The model under review builds one solid part; all positions refer to its coordinate system, in mm. A direction names the side the tool comes from. Round coordinates to 2 decimals unless told otherwise and drop trailing zeros. Loops run counter-clockwise (first coordinate to the right, second up) from the corner with the lowest first, then second, coordinate; pieces in that order, holes last. Notation, with made-up numbers: M -16,-27 L 10,-27 A26 ccw 10,4 Z; hole C -15,21.5 d2. An arc over 180 degrees is marked long. Return JSON: item names as keys, results as strings. Group by question number.
Q1. For faces 4 (the face through (84.51, 2.75, 4.59)), 5 (the face through (1, 0, -1)), 6 (the face through (50.8, 3, -16)), list the 3-axis set-ups (+Z, -Z, +X, -X, +Y, -Y) from which the entire face can be reached by the end or side of a thin tool; tool diameter is ignored.
Q2. Clearance check with a flat-ended pin moving along its axis: pin 1 Ø0.8 at (x, z) = (76.2, 18.72) entering from +Y. State where the tip first meets the part, or that it passes through.
Q3. To check wall thickness, follow line 1 along X through (y, z) = (2.2, -15.5); line 2 along Z through (x, y) = (-0.5, 0.95); line 3 along X through (y, z) = (2.1, 18.5). State the ranges of each line that lie inside material, in increasing order.
Q4. Draft analysis for pull direction X (two halves, no side actions). For faces 1 (the face through (81.235, 2.755, -0.035)), 2 (the face through (1, 5.588, -1)), 3 (the face through (91.61, 2.75, -17.95)), state which applies: pulls with the +X half, pulls with the -X half, needs draft (parallel to the pull), parting line crosses it, or undercut.
Q5. Consider section A-A (x = 44.45). State the section outline as (y, z) points, and give its area (3 significant figures).
Q6. Consider section B-B (z = -38.1). State the section outline as (x, y) points.
Q7. Consider section C-C (y = 1.5). Count the separate pieces of the cut face and the enclosed holes in it, and give its area (3 significant figures).
from build123d import *

# Parameters (mm, degrees)
BOSS_EXTRUDE1_DEPTH             = 5.588
F_1_4_CLEARANCE_HOLE1_D         = 6.35
F_1_4_CLEARANCE_HOLE1_DEPTH     = 5.588
CUT_EXTRUDE1_DEPTH              = 5.588
CUT_EXTRUDE2_REACH              = 7.588
F_4_CLEARANCE_HOLE1_D           = 3.937
F_4_CLEARANCE_HOLE1_DEPTH       = 5.588
CUT_EXTRUDE3_DEPTH              = 5.588
SKETCH15_R                      = 0.635
CUT_EXTRUDE5_DEPTH              = 5.588
MIRROR2_COPY_1_SKETCH_R         = 0.635
MIRROR2_COPY_1_DEPTH            = 5.588
F_10_CLEARANCE_HOLE1_D          = 6.7818
F_10_CLEARANCE_HOLE1_DEPTH      = 5.588
TAP_DRILL_FOR_4_HELICOIL1_D     = 4.064
TAP_DRILL_FOR_4_HELICOIL1_DEPTH = 6.35
TAP_DRILL_FOR_4_HELICOIL1_TIP   = 1.220948778
CUT_EXTRUDE4_REACH              = 7.588


with BuildPart() as part:
    # Sketch1 → Boss-Extrude1 (new body)
    with BuildSketch(Plane(origin=(0, 0, 0), x_dir=(1, 0, 0), z_dir=(0, 1, 0))):
        with BuildLine():
            Line((-101.6, 50.8), (101.6, 50.8))
            Line((101.6, 50.8), (101.6, 7.9375))
            Line((101.6, 7.9375), (89.172371939, 7.9375))
            ThreePointArc((89.172371939, 7.9375), (87.957352042, 7.695817516), (86.927307909, 7.00756403))
            Line((86.927307909, 7.00756403), (82.164807909, 2.24506403))
            ThreePointArc((82.164807909, 2.24506403), (81.234871939, 0), (82.164807909, -2.24506403))
            Line((82.164807909, -2.24506403), (86.927307909, -7.00756403))
            ThreePointArc((86.927307909, -7.00756403), (87.957352042, -7.695817516), (89.172371939, -7.9375))
            Line((89.172371939, -7.9375), (101.6, -7.9375))
            Line((101.6, -7.9375), (101.6, -50.8))
            Line((101.6, -50.8), (-101.6, -50.8))
            Line((-101.6, -50.8), (-101.6, 50.8))
        make_face()
    extrude(amount=BOSS_EXTRUDE1_DEPTH)

    # 1/4 Clearance Hole1
    with Locations(Plane(origin=(0, 5.588, 0), x_dir=(-1, 0, 0), z_dir=(0, 1, 0))):
        with Locations((-88.10625, 38.1), (-88.10625, -38.1), (88.9, 25.4)):
            Hole(F_1_4_CLEARANCE_HOLE1_D / 2, depth=F_1_4_CLEARANCE_HOLE1_DEPTH)

    # Sketch4 → Cut-Extrude1 (cut)
    with BuildSketch(Plane(origin=(0, 5.588, 0), x_dir=(1, 0, 0), z_dir=(0, 1, 0))):
        with BuildLine():
            Line((88.10625, 41.275), (101.6, 41.275))
            Line((101.6, 41.275), (101.6, 34.925))
            Line((101.6, 34.925), (88.10625, 34.925))
            ThreePointArc((88.10625, 34.925), (84.93125, 38.1), (88.10625, 41.275))
        make_face()
    cut_extrude1 = extrude(amount=-CUT_EXTRUDE1_DEPTH, mode=Mode.SUBTRACT)

    # Mirror1: Cut-Extrude1 across plane
    add(cut_extrude1.mirror(Plane.XY), mode=Mode.SUBTRACT)

    # Sketch5 → Cut-Extrude2 (cut, up to next)
    with BuildSketch(Plane(origin=(0, 5.588, 0), x_dir=(1, 0, 0), z_dir=(0, 1, 0)), mode=Mode.PRIVATE) as cut_extrude2_sk1:
        with BuildLine():
            Line((-92.075, -22.225), (-88.9, -22.225))
            ThreePointArc((-88.9, -22.225), (-85.725, -25.4), (-88.9, -28.575))
            Line((-88.9, -28.575), (-92.075, -28.575))
            ThreePointArc((-92.075, -28.575), (-95.25, -25.4), (-92.075, -22.225))
        make_face()
    cut_extrude2_tool1 = extrude(cut_extrude2_sk1.sketch, amount=-CUT_EXTRUDE2_REACH, mode=Mode.PRIVATE) & part.part
    add(cut_extrude2_tool1.solids().sort_by_distance((-90.4875, 5.588, 25.4))[0], mode=Mode.SUBTRACT)

    # #4 Clearance Hole1
    with Locations(Plane(origin=(0, 5.588, 0), x_dir=(-1, 0, 0), z_dir=(0, 1, 0))):
        with Locations((86.36, -43.18), (35.56, -27.94), (35.56, 0), (87.63, 5.08)):
            Hole(F_4_CLEARANCE_HOLE1_D / 2, depth=F_4_CLEARANCE_HOLE1_DEPTH)

    # Sketch9 → Cut-Extrude3 (cut)
    with BuildSketch(Plane(origin=(0, 5.588, 0), x_dir=(1, 0, 0), z_dir=(0, 1, 0))):
        Polygon((-6.0325, 18.7198), (6.0325, 18.7198), (6.35, 18.7198), (12.7, 18.7198), (12.7, 12.7), (6.35, 12.7), (6.0325, 12.7), (-6.0325, 12.7), (-6.35, 12.7), (-12.7, 12.7), (-12.7, 18.7198), (-6.35, 18.7198), align=None)
        Polygon((69.5325, 12.7), (57.4675, 12.7), (57.15, 12.7), (50.8, 12.7), (50.8, 18.7198), (57.15, 18.7198), (57.4675, 18.7198), (69.5325, 18.7198), (69.85, 18.7198), (76.2, 18.7198), (76.2, 12.7), (69.85, 12.7), align=None)
    cut_extrude3 = extrude(amount=-CUT_EXTRUDE3_DEPTH, mode=Mode.SUBTRACT)

    # Sketch15 → Cut-Extrude5 (cut)
    with BuildSketch(Plane(origin=(0, 5.588, 0), x_dir=(1, 0, 0), z_dir=(0, 1, 0))):
        with Locations((-12.7, 18.7198)):
            Circle(SKETCH15_R)
        with Locations((12.7, 18.7198)):
            Circle(SKETCH15_R)
        with Locations((12.7, 12.7)):
            Circle(SKETCH15_R)
        with Locations((-12.7, 12.7)):
            Circle(SKETCH15_R)
    cut_extrude5 = extrude(amount=-CUT_EXTRUDE5_DEPTH, mode=Mode.SUBTRACT)

    # Mirror3: Cut-Extrude5 across plane
    add(cut_extrude5.mirror(Plane.ZY.offset(-31.75)), mode=Mode.SUBTRACT)

    # Mirror2: Cut-Extrude3, Cut-Extrude5 across plane
    add(cut_extrude3.mirror(Plane.XY), mode=Mode.SUBTRACT)
    add(cut_extrude5.mirror(Plane.XY), mode=Mode.SUBTRACT)

    # Mirror2 copy 1 sketch → Mirror2 copy 1 (cut)
    with BuildSketch(Plane(origin=(63.5, 5.588, 0), x_dir=(-1, 0, 0), z_dir=(0, 1, 0))):
        with Locations((-12.7, 18.7198)):
            Circle(MIRROR2_COPY_1_SKETCH_R)
        with Locations((12.7, 18.7198)):
            Circle(MIRROR2_COPY_1_SKETCH_R)
        with Locations((12.7, 12.7)):
            Circle(MIRROR2_COPY_1_SKETCH_R)
        with Locations((-12.7, 12.7)):
            Circle(MIRROR2_COPY_1_SKETCH_R)
    extrude(amount=-MIRROR2_COPY_1_DEPTH, mode=Mode.SUBTRACT)

    # #10 Clearance Hole1
    with Locations(Plane(origin=(0, 5.588, 0), x_dir=(-1, 0, 0), z_dir=(0, 1, 0))):
        with Locations((-19.05, 0), (-44.45, 0)):
            Hole(F_10_CLEARANCE_HOLE1_D / 2, depth=F_10_CLEARANCE_HOLE1_DEPTH)

    # Tap Drill for #4 Helicoil1
    with Locations(Plane(origin=(0, 5.588, 0), x_dir=(1, 0, 0), z_dir=(0, 1, 0))):
        with Locations((93.4847, 18.7325), (83.9597, 18.7325)):
            Hole(TAP_DRILL_FOR_4_HELICOIL1_D / 2, depth=TAP_DRILL_FOR_4_HELICOIL1_DEPTH)
            with Locations((0, 0, -(TAP_DRILL_FOR_4_HELICOIL1_DEPTH + TAP_DRILL_FOR_4_HELICOIL1_TIP / 2))):  # 118° drill point
                Cone(0, TAP_DRILL_FOR_4_HELICOIL1_D / 2, TAP_DRILL_FOR_4_HELICOIL1_TIP, mode=Mode.SUBTRACT)

    # Sketch14 → Cut-Extrude4 (cut, up to next)
    with BuildSketch(Plane(origin=(0, 5.588, 0), x_dir=(1, 0, 0), z_dir=(0, 1, 0)), mode=Mode.PRIVATE) as cut_extrude4_sk1:
        with BuildLine():
            Line((-88.9, -22.225), (-82.55, -22.225))
            ThreePointArc((-82.55, -22.225), (-79.375, -25.4), (-82.55, -28.575))
            Line((-82.55, -28.575), (-88.9, -28.575))
            ThreePointArc((-88.9, -28.575), (-85.725, -25.4), (-88.9, -22.225))
        make_face()
    cut_extrude4_tool1 = extrude(cut_extrude4_sk1.sketch, amount=-CUT_EXTRUDE4_REACH, mode=Mode.PRIVATE) & part.part
    add(cut_extrude4_tool1.solids().sort_by_distance((-83.231361, 5.588, 25.4))[0], mode=Mode.SUBTRACT)


solid = part.part
Values:
{
 "1": {"face 4": "+X, +Y, -Y", "face 5": "+Z, -Z, +X, -X, -Y", "face 6": "+Y, -Y"},
 "2": {"pin 1": "passes through"},
 "3": {"line 1": "x = -101.6 to -12.7, 12.7 to 50.8, 76.2 to 101.6", "line 2": "z = -50.8 to -18.72, -12.7 to 12.7, 18.72 to 50.8", "line 3": "x = -101.6 to -13.3, 13.3 to 50.2, 76.8 to 101.6"},
 "4": {"face 1": "pulls with the +X half", "face 2": "needs draft", "face 3": "undercut"},
 "5": {"outline": "M 0,-50.8 L 5.59,-50.8 L 5.59,-3.39 L 0,-3.39 Z; M 0,3.39 L 5.59,3.39 L 5.59,50.8 L 0,50.8 Z", "area": "530 mm2"},
 "6": {"outline": "M -101.6,0 L 84.93,0 L 84.93,5.59 L -101.6,5.59 Z"},
 "7": {"separate pieces": "1", "enclosed holes": "13", "area": "19,300 mm2"}
}
